Check sheet for the modelled part. Datum: model origin and axes. Units: mm. A direction names the side the tool comes from. Round coordinates to 2 decimals unless told otherwise and drop trailing zeros. Write each loop counter-clockwise with the first axis right and the second up, starting at its lowest first coordinate (ties: lowest second). Pieces come first, ordered by that corner, then holes. Notation, with made-up numbers: (72, -28) - (93, -28) arc R15 cw to (93, -17) - close; hole circle Ø1 at (-9, -15.5). An arc over 180 degrees is marked (long way). Answer as a JSON object with one key per item and string values. Group by question number.
Item 1: Sectioned sample at C-C on x = 22. Record the boundary of the cut face in (y, z).
Item 2: Release check for a two-part mould opening along X. For faces 1 (the cylindrical face through (-74.064, 40.413, 10.14)), 2 (the cylindrical face through (0.84, -28.93, 1.5)), 3 (the flat face through (-17, -34, 0)) record: pulls with the +X half, pulls with the -X half, needs draft (parallel to the pull), parting line crosses it, or undercut.
Item 3: Sectioned sample at D-D on x = -65.5. Record the boundary of the cut face in (y, z).
Item 4: Thickness scan on line 1 (Y direction, x = 46, z = 15.5); line 2 (X direction, y = 8.5, z = 3.5); line 3 (Y direction, x = -11, z = 7.25). Record the ranges inside material, lowest first.
Item 5: Sectioned sample at B-B on y = 3. Record the boundary of the cut face in (x, z), plus the area to 3 significant figures.
Item 6: Sectioned sample at A-A on x = 44.5. Record the boundary of the cut face in (y, z), plus the area to 3 significant figures.
Item 7: Gauge pin test, flat ends, axial feed: P1, Ø6, axis at x = -18.5, z = 7.5, coming from the -Y side; P2, Ø2, axis at x = -70, z = 10.5, coming from the -Y side; P3, Ø12, axis at x = -37, y = -61.5, coming from the -Z side; P4, Ø6, axis at y = -51.5, z = 12, coming from the -X side. Record the tip position at first contact, or that the pin passes through.
Item 8: Set-up check for faces 4 (the flat face through (-75, -2, 10)), 5 (the cylindrical face through (-14.788, 31.488, 10.14)), 6 (the cylindrical face through (-74.3, -87.046, 9.86)), 7 (the flat face through (71, -42.5, 10)), 8 (the flat face through (-71, -42.5, 10)): record each of +Z, -Z, +X, -X, +Y, -Y from which the full face is reachable in a straight line by a thin tool's end or side.
```python
from build123d import *

# Parameters (mm, degrees)
F0_W     = 120
F0_H     = 55
F1_DEPTH = 20
F2_R     = 5
F4_DEPTH = 20.001


with BuildPart() as f1:
    # F0 (on Top) → F1 (new body)
    with BuildSketch(Plane.XY):
        Polygon((75, -42.5), (75, 42.5), (-75, 42.5), (-75, -42.5), (-67.5, -42.5), (-57.5, -42.5), (-5, -42.5), (5, -42.5), (57.5, -42.5), (67.5, -42.5), align=None)
        Rectangle(F0_W, F0_H, mode=Mode.SUBTRACT)
        with BuildLine():
            Line((67.5, -68.693042), (67.5, -42.5))
            Line((67.5, -42.5), (57.5, -42.5))
            Line((57.5, -42.5), (57.5, -68.693042))
            ThreePointArc((57.5, -68.693042), (49.808453, -77.539779), (39.978338, -71.152801))
            ThreePointArc((39.978338, -71.152801), (33.309749, -67.591487), (29.962853, -74.370228))
            ThreePointArc((29.962853, -74.370228), (51.069883, -86.993343), (67.5, -68.693042))
        make_face()
        with BuildLine():
            Line((-57.5, -42.5), (-67.5, -42.5))
            Line((-67.5, -42.5), (-67.5, -68.693042))
            ThreePointArc((-67.5, -68.693042), (-75.191547, -77.539779), (-85.021662, -71.152801))
            ThreePointArc((-85.021662, -71.152801), (-91.690251, -67.591487), (-95.037147, -74.370228))
            ThreePointArc((-95.037147, -74.370228), (-73.930117, -86.993343), (-57.5, -68.693042))
            Line((-57.5, -68.693042), (-57.5, -42.5))
        make_face()
        with BuildLine():
            Line((5, -68.693042), (5, -42.5))
            Line((5, -42.5), (-5, -42.5))
            Line((-5, -42.5), (-5, -68.693042))
            ThreePointArc((-5, -68.693042), (-12.691547, -77.539779), (-22.521662, -71.152801))
            ThreePointArc((-22.521662, -71.152801), (-29.190251, -67.591487), (-32.537147, -74.370228))
            ThreePointArc((-32.537147, -74.370228), (-11.430117, -86.993343), (5, -68.693042))
        make_face()
    extrude(amount=F1_DEPTH)

    # F2
    f2_edges = [f1.edges().sort_by_distance(p)[0] for p in [
        (0, 42.5, 20),
        (0, 42.5, 0),
        (-75, 42.5, 10),
        (75, 42.5, 10),
        (0, -27.5, 0),
        (0, -27.5, 20),
    ]]
    fillet(f2_edges, radius=F2_R)

    # F3 (on face) → F4 (cut, through all)
    with BuildSketch(Plane.XY.offset(20)):
        with BuildLine():
            Line((-59.415153, 27.492821), (-30, 27.131766))
            ThreePointArc((-30, 27.131766), (-44.656341, 31.486476), (-59.415153, 27.492821))
        make_face()
        with BuildLine():
            ThreePointArc((59.415153, 27.492821), (44.656341, 31.486476), (30, 27.131766))
            Line((30, 27.131766), (59.415153, 27.492821))
        make_face()
        with BuildLine():
            ThreePointArc((30, 27.131766), (15, 31.488585), (0, 27.131766))
            Line((0, 27.131766), (30, 27.131766))
        make_face()
        with BuildLine():
            ThreePointArc((0, 27.131766), (-15, 31.488585), (-30, 27.131766))
            Line((-30, 27.131766), (0, 27.131766))
        make_face()
    extrude(amount=-F4_DEPTH, mode=Mode.SUBTRACT)


solid = f1.part
```
Completed:
{
 "1": {"outline": "(-42.5, 0) - (-32.5, 0) arc R5 ccw to (-27.5, 5) - (-27.5, 15) arc R5 ccw to (-32.5, 20) - (-42.5, 20) - close; (30.6, 0) - (37.5, 0) arc R5 ccw to (42.5, 5) - (42.5, 15) arc R5 ccw to (37.5, 20) - (30.6, 20) - close"},
 "2": {"face 1": "pulls with the -X half", "face 2": "undercut", "face 3": "needs draft"},
 "3": {"outline": "(-83.55, 0) - (37.5, 0) arc R5 ccw to (42.5, 5) - (42.5, 15) arc R5 ccw to (37.5, 20) - (-83.55, 20) - close"},
 "4": {"line 1": "-87.09 to -77.25, -42.5 to -27.53, 31.47 to 42.47", "line 2": "-75 to -60, 60 to 75", "line 3": "-86.92 to -77.13, -42.5 to -27.5, 31.2 to 42.5"},
 "5": {"outline": "(-75, 0) - (-60, 0) - (-60, 20) - (-75, 20) - close; (60, 0) - (75, 0) - (75, 20) - (60, 20) - close", "area": "600 mm²"},
 "6": {"outline": "(-86.86, 0) - (-76.65, 0) - (-76.65, 20) - (-86.86, 20) - close; (-42.5, 0) - (-32.5, 0) arc R5 ccw to (-27.5, 5) - (-27.5, 15) arc R5 ccw to (-32.5, 20) - (-42.5, 20) - close; (31.48, 0) - (37.5, 0) arc R5 ccw to (42.5, 5) - (42.5, 15) arc R5 ccw to (37.5, 20) - (31.48, 20) - close", "area": "703 mm²"},
 "7": {"P1": "y = -87.17", "P2": "y = -86.31", "P3": "through", "P4": "x = -67.5"},
 "8": {"face 4": "+Z, -Z, -X, +Y", "face 5": "+Z, -Z", "face 6": "+Z, -Z, -Y", "face 7": "+Z, -Z, +X, -Y", "face 8": "+Z, -Z, -X"}
}
